Part model, mm, in its own coordinate system. A direction names the side the tool comes from. Give positions to 0.01 mm unless a question says otherwise; leave off trailing zeros. Write each loop counter-clockwise with the first axis right and the second up, starting at its lowest first coordinate (ties: lowest second). Pieces come first, ordered by that corner, then holes.
```python
from build123d import *

# Parameters (mm, degrees)
BASPROSKE_W         = 10
BASPROSKE_H         = 7.5
TOOTHCUT_DEPTH      = 15.577379737
TEETHCUTS_COUNT     = 13
TEETHCUTS_ANGLE     = 332.307692308
BORSKE_R            = 0.4
BORE_DEPTH          = 50.0000508
SKETCH1_R           = 9.25
BOSS_EXTRUDE1_DEPTH = 3
SKETCH6_R           = 0.5
CUT_EXTRUDE1_DEPTH  = 2
CIRPATTERN1_COUNT   = 6


with BuildPart() as part:
    # BasProSke → Base-Revolve (revolve)
    with BuildSketch(Plane(origin=(0, 0, 0), x_dir=(1, 0, 0), z_dir=(0, 1, 0)), mode=Mode.PRIVATE) as base_revolve_sk:
        with Locations((5, 3.75)):
            Rectangle(BASPROSKE_W, BASPROSKE_H)
    revolve(base_revolve_sk.sketch.rotate(Axis((-10, 0, 0), (1, 0, 0)), 180), axis=Axis((-10, 0, 0), (1, 0, 0)))

    # TooCutSke → ToothCut (cut, through all)
    with BuildSketch(Plane(origin=(0, 0, 0), x_dir=(0, 0, -1), z_dir=(1, 0, 0))):
        with BuildLine():
            ThreePointArc((0.550489643, 5.220053846), (0, 5.249), (-0.550489643, 5.220053846))
            ThreePointArc((-0.550489643, 5.220053846), (-0.834571714, 6.414617604), (-1.635166801, 7.345602405))
            ThreePointArc((-1.635166801, 7.345602405), (0, 7.5254), (1.635166801, 7.345602405))
            ThreePointArc((1.635166801, 7.345602405), (0.834571714, 6.414617604), (0.550489643, 5.220053846))
        make_face()
    toothcut = extrude(amount=TOOTHCUT_DEPTH, mode=Mode.SUBTRACT)

    # TeethCuts: ToothCut ×13 about axis
    teethcuts_axis = Axis((-10, 0, 0), (1, 0, 0))
    for i in range(1, TEETHCUTS_COUNT):
        add(toothcut.rotate(teethcuts_axis, i * TEETHCUTS_ANGLE / (TEETHCUTS_COUNT - 1)), mode=Mode.SUBTRACT)

    # BorSke → Bore (cut, symmetric)
    with BuildSketch(Plane(origin=(0, 0, 0), x_dir=(0, 0, -1), z_dir=(1, 0, 0))):
        with Locations(Location((0, 0, 0), (0, 0, 180))):
            Circle(BORSKE_R)
    extrude(amount=BORE_DEPTH, both=True, mode=Mode.SUBTRACT)

    # Sketch1 → Boss-Extrude1 (add)
    with BuildSketch(Plane.ZY):
        Circle(SKETCH1_R)
    extrude(amount=BOSS_EXTRUDE1_DEPTH)

    # Sketch6 → Cut-Extrude1 (cut)
    with BuildSketch(Plane.ZY.offset(3)):
        with Locations((-8.01665008, -1.724332186)):
            Circle(SKETCH6_R)
    cut_extrude1 = extrude(amount=-CUT_EXTRUDE1_DEPTH, mode=Mode.SUBTRACT)

    # CirPattern1: Cut-Extrude1 ×6 about axis
    cirpattern1_axis = Axis((0, 0, 0), (1, 0, 0))
    for i in range(1, CIRPATTERN1_COUNT):
        add(cut_extrude1.rotate(cirpattern1_axis, i * 360 / CIRPATTERN1_COUNT), mode=Mode.SUBTRACT)


solid = part.part
```
1) Saw through at A-A, the plane y = 4. Write the cut outline in (x, z), then the cut area to 3 significant figures.
Answers follow:
outline: (-3, -8.34) - (0, -8.34) - (0, -4.59) - (10, -4.59) - (10, 4.59) - (0, 4.59) - (0, 8.34) - (-3, 8.34) - close
area: 142 mm2
2) 3-axis set-ups, long thin cutter, end or side, ignore diameter. For faces 1 (the face through (4.93, -3.055, -5.702)), 2 (the face through (4.93, -3.03, 5.68)), 3 (the face through (-2.014, 5.743, -5.133)), 4 (the face through (4.93, -6.029, 2.346)): which of +Z, -Z, +X, -X, +Y, -Y reach the whole face in a straight line?
Answers follow:
face 1: -Z, +X
face 2: +Z, +X
face 3: -X
face 4: +X, -Y
3) Pin check, flat tips, straight feed: pin 1 Ø0.5 at (y, z) = (6, -5.5) entering from -X; pin 2 Ø6 at (y, z) = (7, -7) entering from -X; pin 3 Ø3 at (x, z) = (5, 7) entering from -Y; pin 4 Ø1 at (x, z) = (5, -3) entering from +Y. Stop position of each tip, or through.
Answers follow:
pin 1: stops at x = -1
pin 2: stops at x = -3
pin 3: stops at y = -4.43
pin 4: stops at y = 5.12
4) Wall check: L1, parallel to Z at x = 6.5, y = 4.5; L2, parallel to Y at x = 6.75, z = 6; L3, parallel to Y at x = 2.5, z = 0. Give the ranges that are in metal, low to high.
Answers follow:
L1: z = -4.89 to -2.99, -2.7 to 2.7, 2.99 to 4.89
L2: y = -4.42 to -3.46, -1.51 to 0.07, 1.44 to 2.98
L3: y = -7.5 to -0.4, 0.4 to 5.25
